Verification items for this drawing (mm, ordinates from the low corner). A direction names the side the tool comes from. Round coordinates to 2 decimals unless told otherwise and drop trailing zeros. Loops run counter-clockwise (first coordinate to the right, second up) from the corner with the lowest first, then second, coordinate; pieces in that order, holes last. Notation, with made-up numbers: (16, 75.5) - (44, 75.5) arc R20 cw to (44, 82.5) - close; hole circle Ø11 at (-8, 89.5). An arc over 180 degrees is marked (long way). Answer in a Markdown table with one row per item. Add a question column.
(1) Thickness scan on line 1 along Z through (x, y) = (92.5, 11); line 2 along Z through (x, y) = (24.5, 7) (1 decimal); line 3 along Z through (x, y) = (48, 6.5). Record the ranges inside material, lowest first.
(2) Cross-section at A-A on z = 64.5. Enter the section's corners in (x, y).
(3) Mould release check, pull along X, two halves, no side actions. Record for the marked faces 1, 2, 3 and 4: +X half, -X half, draft (parallel to the pull), parting line (faces both ways), or undercut.
(4) Access from +Z, -Z, +X, -X, +Y, -Y to the whole of each face (thin tool, end or side, straight path). Record for the marked faces 5, 6 and 7.
(5) Gauge pin test, flat ends, axial feed: pin 1 (4 mm diameter, centred on x = 88, y = 1.5, fed in from +Z) (1 decimal); pin 2 (4 mm diameter, centred on y = 11, z = 81.5, fed in from -X); pin 3 (1.5 mm diameter, centred on x = 33.5, y = 10, fed in from +Z). Record the tip position at first contact, or that the pin passes through.
(6) Cross-section at B-B on x = 19.5. Enter the section's corners in (y, z).
(7) Cross-section at C-C on y = 8.5. Enter the section's corners in (x, z) (1 decimal).
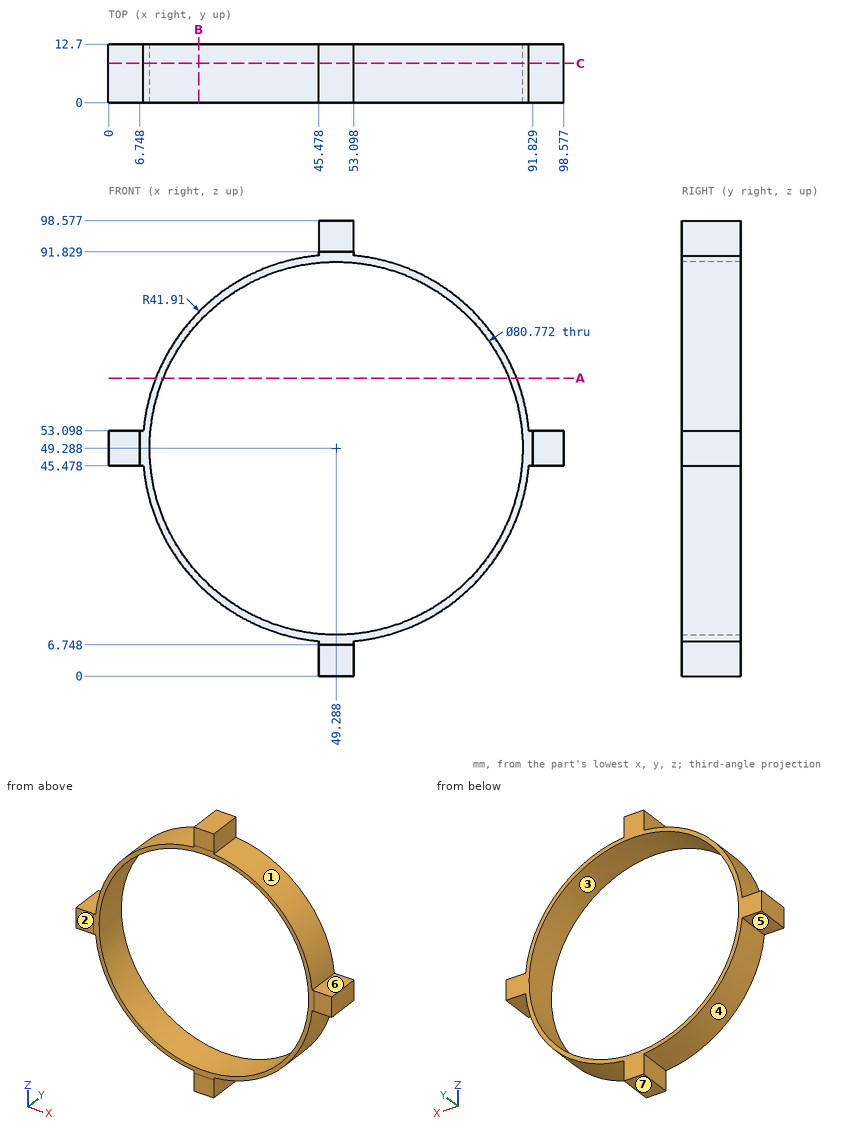
Answers:
| question | item | result |
|---|---|---|
| 1 | line 1 | z = 45.48 to 53.1 |
| 1 | line 2 | z = 15.5 to 17.4, 81.2 to 83.1 |
| 1 | line 3 | z = 0 to 8.92, 89.65 to 98.58 |
| 2 | outline | (10.24, 0) - (11.88, 0) - (11.88, 12.7) - (10.24, 12.7) - close; (86.7, 0) - (88.34, 0) - (88.34, 12.7) - (86.7, 12.7) - close |
| 3 | face 1 | +X half |
| 3 | face 2 | draft |
| 3 | face 3 | undercut |
| 3 | face 4 | -X half |
| 4 | face 5 | -Z, -X, +Y, -Y |
| 4 | face 6 | +Z, +X, +Y, -Y |
| 4 | face 7 | -Z, +X, -X, +Y, -Y |
| 5 | pin 1 | stops at z = 69.5 |
| 5 | pin 2 | stops at x = 20.24 |
| 5 | pin 3 | stops at z = 88.41 |
| 6 | outline | (0, 19.81) - (12.7, 19.81) - (12.7, 22.02) - (0, 22.02) - close; (0, 76.56) - (12.7, 76.56) - (12.7, 78.77) - (0, 78.77) - close |
| 7 | outline | (0, 45.5) - (7.6, 45.5) arc R41.9 ccw to (45.5, 7.6) - (45.5, 0) - (53.1, 0) - (53.1, 7.6) arc R41.9 ccw to (91, 45.5) - (98.6, 45.5) - (98.6, 53.1) - (91, 53.1) arc R41.9 ccw to (53.1, 91) - (53.1, 98.6) - (45.5, 98.6) - (45.5, 91) arc R41.9 ccw to (7.6, 53.1) - (0, 53.1) - close; hole circle Ø80.8 at (49.3, 49.3) |
